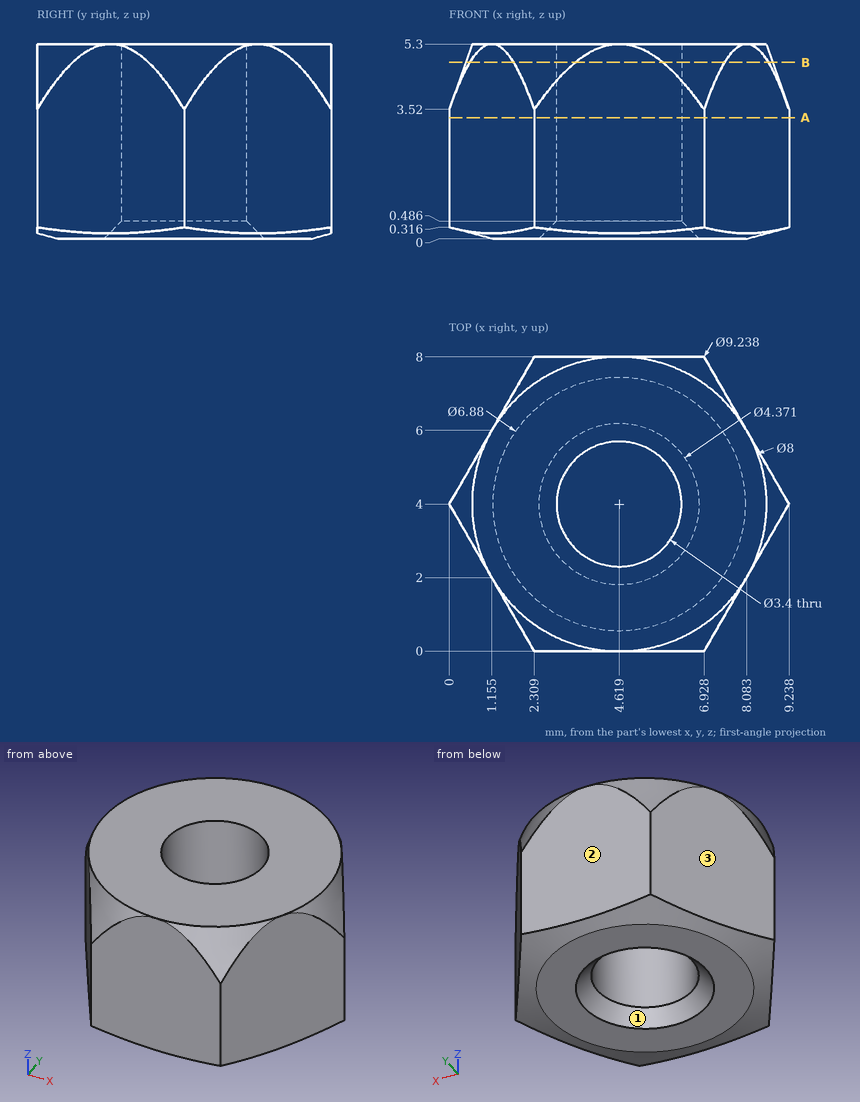
Job drawing, mm, ordinate dimensions from the low corner. One solid piece. Give positions to 0.01 mm unless a question says otherwise; leave off trailing zeros. Loops run counter-clockwise (first coordinate to the right, second up) from the corner with the lowest first, then second, coordinate; pieces in that order, holes last. Notation, with made-up numbers: M 36,24 L 67,24 A12 ccw 67,31 Z; hole C 85.5,89 d7. An arc over 180 degrees is marked long. Return JSON: item names as keys, results as strings.
1) Drill centre lines: line 1 (X direction, y = 2, z = 0.85) (1 decimal); line 2 (X direction, y = 5.25, z = 3.15) (1 decimal); line 3 (Y direction, x = 3.5, z = 3.45). Where is each one in solid material? Low to high.
Calculated:
{"line 1": "x = 1.2 to 8.1", "line 2": "x = 0.7 to 3.5, 5.8 to 8.5", "line 3": "y = 0 to 2.72, 5.28 to 8"}
2) Flat gauge pin, fed straight in: pin 1 Ø1 at (y, z) = (5.5, 3.5) entering from -X. Where does the tip first touch, or does it go through?
Calculated:
{"pin 1": "stops at x = 0.58"}
3) Saw through at B-B, the plane z = 4.8. List the corners of the cut face in (x, y).
Calculated:
{"outline": "M 0.56,3.03 L 1.75,0.97 A4.17 ccw 3.43,0 L 5.81,0 A4.17 ccw 7.49,0.97 L 8.68,3.03 A4.17 ccw 8.68,4.97 L 7.49,7.03 A4.17 ccw 5.81,8 L 3.43,8 A4.17 ccw 1.75,7.03 L 0.56,4.97 A4.17 ccw Z; hole C 4.62,4 d3.4"}
4) Saw through at A-A, the plane z = 3.3. List the corners of the cut face in (x, y).
Calculated:
{"outline": "M 0,4 L 2.31,0 L 6.93,0 L 9.24,4 L 6.93,8 L 2.31,8 Z; hole C 4.62,4 d3.4"}
5) Pull direction X, two halves, no side cores. Call the marked faces 1, 2 and 3: released by +X, released by -X, zero draft, split by the parting line, or undercut.
Calculated:
{"face 1": "undercut", "face 2": "zero draft", "face 3": "released by -X"}
